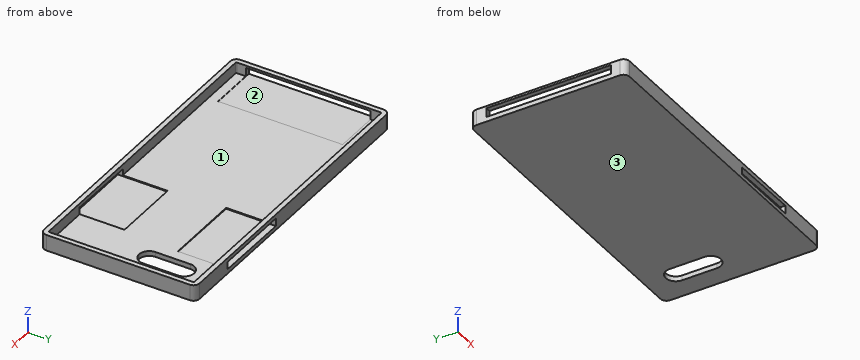
from build123d import *

# Parameters (mm, degrees)
F0_W      = 157
F0_H      = 78
F1_DEPTH  = 8
F2_R      = 3
F3_T      = -2.5
F5_DEPTH  = 25
F7_W      = 62.540936
F7_H      = 4.507454
F8_DEPTH  = 25
F11_DEPTH = 25
F12_DEPTH = 25


with BuildPart() as f1:
    # F0 (on Top) → F1 (new body)
    with BuildSketch(Plane.XY):
        with Locations((78.5, 39)):
            Rectangle(F0_W, F0_H)
    extrude(amount=F1_DEPTH)

    # F2
    f2_edges = [f1.edges().sort_by_distance(p)[0] for p in [
        (157, 0, 4),
        (157, 78, 4),
        (0, 78, 4),
        (0, 0, 4),
    ]]
    fillet(f2_edges, radius=F2_R)

    # F3
    f3_openings = [f1.faces().sort_by_distance(p)[0] for p in [
        (78.5, 39, 8),
    ]]
    offset(amount=F3_T, openings=f3_openings)

    # F4 (on face) → F5 (cut)
    with BuildSketch(Plane.XY.offset(2.5)):
        with BuildLine():
            ThreePointArc((146.744221, 62.751937), (145.279755, 66.287471), (141.744221, 67.751937))
            Line((141.744221, 67.751937), (141.66825, 67.751937))
            ThreePointArc((141.66825, 67.751937), (138.132716, 66.287471), (136.66825, 62.751937))
            Line((136.66825, 62.751937), (136.66825, 45.115006))
            ThreePointArc((136.66825, 45.115006), (138.132716, 41.579472), (141.66825, 40.115006))
            Line((141.66825, 40.115006), (141.744221, 40.115006))
            ThreePointArc((141.744221, 40.115006), (145.279755, 41.579472), (146.744221, 45.115006))
            Line((146.744221, 45.115006), (146.744221, 62.751937))
        make_face()
    extrude(amount=-F5_DEPTH, mode=Mode.SUBTRACT)

    # F7 (on face) → F8 (cut)
    with BuildSketch(Plane(origin=(0, 0, 0), x_dir=(0, -1, 0), z_dir=(-1, 0, 0))):
        with Locations((-38.633815, 4.610173)):
            Rectangle(F7_W, F7_H)
    extrude(amount=-F8_DEPTH, mode=Mode.SUBTRACT)

    # F10 (on face) → F11 (cut)
    with BuildSketch(Plane.XZ):
        Polygon((129.16705, 6.068889), (94.259493, 5.586785), (94.259493, 2.000924), (129.16705, 2.000924), align=None)
    extrude(amount=-F11_DEPTH, mode=Mode.SUBTRACT)

    # F9 (on face) → F12 (cut)
    with BuildSketch(Plane(origin=(0, 78, 0), x_dir=(-1, 0, 0), z_dir=(0, 1, 0))):
        Polygon((-131.193131, 2.239336), (-92.129149, 1.990521), (-92.129149, 5.971564), (-131.193131, 5.971564), align=None)
    extrude(amount=-F12_DEPTH, mode=Mode.SUBTRACT)


solid = f1.part
Check sheet for the modelled part. Datum: model origin and axes. Units: mm. Face numbers are marked on the shaded views. Round coordinates to 2 decimals unless told otherwise and drop trailing zeros. Loops run counter-clockwise (first coordinate to the right, second up) from the corner with the lowest first, then second, coordinate; pieces in that order, holes last. Notation, with made-up numbers: (41, -3) -> (51, -3) arc R11 cw to (51, 2) -> close; hole circle Ø10 at (-22.75, 41.25). An arc over 180 degrees is marked (long way). Put each result on its own line as item: value. Start each with the question number.
1. Gauge pin test, flat ends, axial feed: pin 1 (3 mm diameter, centred on y = 33.5, z = 5, fed in from -X); pin 2 (0.5 mm diameter, centred on x = 117, z = 2.5, fed in from -Y); pin 3 (5 mm diameter, centred on x = 73.5, y = 36, fed in from +Z). Record the tip position at first contact, or that the pin passes through.
2. Section check A-A (z = 4). Enter the section's corners in (x, y), plus the area to 3 significant figures.
3. Section check D-D (y = 71.5). Enter the section's corners in (x, z), plus the area to 3 significant figures.
4. Section check C-C (x = 103.5). Enter the section's corners in (y, z), plus the area to 3 significant figures.
5. Scan lines: probe 1 along Y at (x, z) = (129.5, 6.25); probe 2 along X at (y, z) = (57, 1.5); probe 3 along X at (y, z) = (74, 4.25). Record each from-to range of solid material in increasing order.
6. Section check B-B (y = 31.5). Enter the section's corners in (x, z).
7. Draft check along Y on the marked faces 1, 2 and 3. Enter one of: +Y half, -Y half, draft (parallel to the pull), parting line (faces both ways), or undercut.
Findings:
1. pin 1: stops at x = 154.5
1. pin 2: stops at y = 25
1. pin 3: stops at z = 2.5
2. outline: (0, 3) arc R3 ccw to (3, 0) -> (94.26, 0) -> (94.26, 2.5) -> (3, 2.5) arc R0.5 cw to (2.5, 3) -> (2.5, 7.36) -> (0, 7.36) -> close; (0, 69.9) -> (2.5, 69.9) -> (2.5, 75) arc R0.5 cw to (3, 75.5) -> (92.13, 75.5) -> (92.13, 78) -> (3, 78) arc R3 ccw to (0, 75) -> close; (129.17, 0) -> (154, 0) arc R3 ccw to (157, 3) -> (157, 75) arc R3 ccw to (154, 78) -> (131.19, 78) -> (131.19, 75.5) -> (154, 75.5) arc R0.5 cw to (154.5, 75) -> (154.5, 3) arc R0.5 cw to (154, 2.5) -> (129.17, 2.5) -> close
2. area: 801 mm^2
3. outline: (0, 0) -> (157, 0) -> (157, 8) -> (154.5, 8) -> (154.5, 2.5) -> (131.19, 2.5) -> (131.19, 2.24) -> (92.13, 1.99) -> (92.13, 2.5) -> (2.5, 2.5) -> (2.5, 8) -> (0, 8) -> close
3. area: 405 mm^2
4. outline: (0, 0) -> (78, 0) -> (78, 2.06) -> (53, 2.06) -> (53, 2.5) -> (25, 2.5) -> (25, 2) -> (0, 2) -> close; (0, 5.71) -> (2.5, 5.71) -> (2.5, 8) -> (0, 8) -> close; (75.5, 5.97) -> (78, 5.97) -> (78, 8) -> (75.5, 8) -> close
4. area: 182 mm^2
5. probe 1: y = 0 to 2.5, 75.5 to 78
5. probe 2: x = 0 to 136.67, 146.74 to 157
5. probe 3: x = 0 to 2.5, 154.5 to 157
6. outline: (0, 0) -> (157, 0) -> (157, 8) -> (154.5, 8) -> (154.5, 2.5) -> (25, 2.5) -> (25, 2.36) -> (0, 2.36) -> close; (0, 6.86) -> (2.5, 6.86) -> (2.5, 8) -> (0, 8) -> close
7. face 1: undercut
7. face 2: undercut
7. face 3: draft
